Answer from the drawing. Dimensions are ordinates in mm from the lowest x, y and z of the part. Give positions to 0.01 mm unless a question says otherwise; leave off trailing zeros. Write each loop counter-clockwise with the first axis right and the second up, starting at its lowest first coordinate (ties: lowest second). Pieces come first, ordered by that corner, then holes. Notation, with made-up numbers: M 27.25,-16.5 L 69.25,-16.5 A28 ccw 69.25,22.5 Z; hole C -21,72.5 d10. An arc over 180 degrees is marked long. Put each result on its own line as item: value.
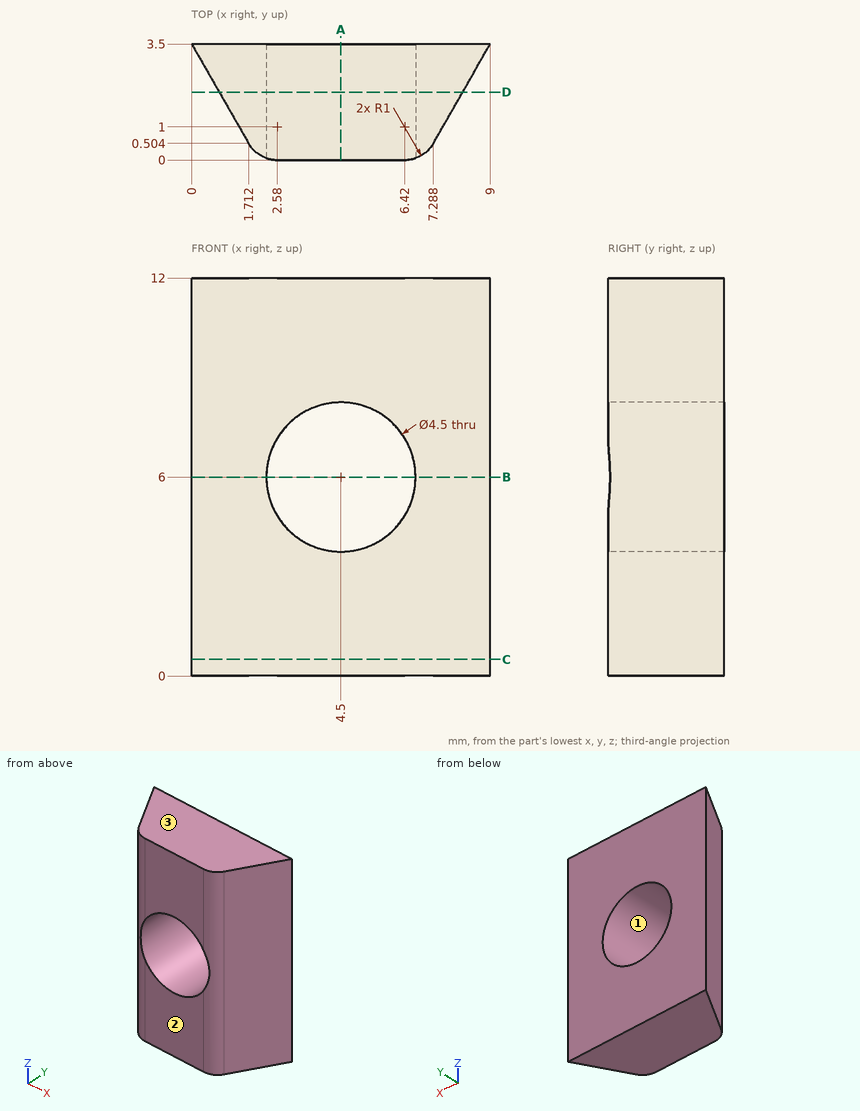
(1) Section B-B on z = 6 is taken. Determine the outline of the cut face in (x, y).
Result:
outline: M 0,3.5 L 1.71,0.5 A1 ccw 2.25,0.06 L 2.25,3.5 Z; M 6.75,0.06 A1 ccw 7.29,0.5 L 9,3.5 L 6.75,3.5 Z
(2) Given pin 1 Ø3 at (x, z) = (8, 4) entering from -Y, flat-ended and moving along its own axis, determine where the tip first touches the part or whether it passes through.
Result:
pin 1: stops at y = 0
(3) Section C-C on z = 0.5 is taken. Determine the outline of the cut face in (x, y).
Result:
outline: M 0,3.5 L 1.71,0.5 A1 ccw 2.58,0 L 6.42,0 A1 ccw 7.29,0.5 L 9,3.5 Z
(4) Section A-A on x = 4.5 is taken. Determine the outline of the cut face in (y, z).
Result:
outline: M 0,0 L 3.5,0 L 3.5,3.75 L 0,3.75 Z; M 0,8.25 L 3.5,8.25 L 3.5,12 L 0,12 Z
(5) Straight lines are drawn through the part: line 1 along Z through (x, y) = (4.5, 2.55); line 2 along Y through (x, z) = (2.5, 11); line 3 along Z through (x, y) = (3.75, 2.45). For each, find the intervals that lie inside material, in ascending order. Write a range as from..to.
Result:
line 1: z = 0..3.75, 8.25..12
line 2: y = 0..3.5
line 3: z = 0..3.88, 8.12..12
(6) For a pull along Z with two mould halves and no side action, classify the marked faces 1, 2 and 3 as +Z half, -Z half, draft (parallel to the pull), parting line (faces both ways), or undercut.
Result:
face 1: undercut
face 2: draft
face 3: +Z half
(7) Section D-D on y = 2.05 is taken. Determine the outline of the cut face in (x, z).
Result:
outline: M 0.83,0 L 8.17,0 L 8.17,12 L 0.83,12 Z; hole C 4.5,6 d4.5
